Answer from the drawing. Dimensions are ordinates in mm from the lowest x, y and z of the part. A direction names the side the tool comes from. Coordinates: 2 decimals unless noted, no trailing zeros. Write each loop counter-clockwise with the first axis right and the second up, starting at its lowest first coordinate (ties: lowest second). Pieces come first, ordered by that corner, then holes. Notation, with made-up numbers: (-39.75, -35) - (-34.75, -35) arc R15 cw to (-34.75, -24) - close; hole circle Ø10 at (78, 9.5). An arc over 180 degrees is marked (long way). Use a Markdown table: item, result.
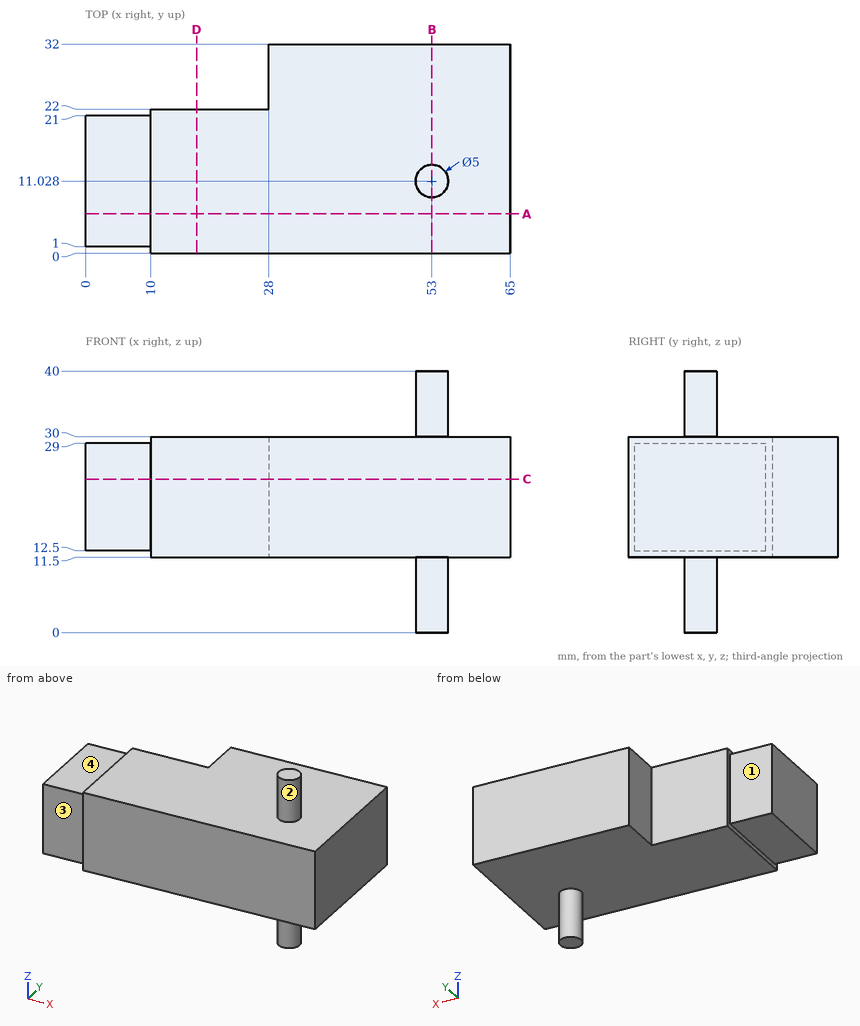
(1) A cutting plane is placed at C-C, the plane z = 23.5. Write down the section's boundary in (x, y), and give its area (3 significant figures).
Report:
| item | result |
|---|---|
| outline | (0, 1) - (10, 1) - (10, 0) - (65, 0) - (65, 32) - (28, 32) - (28, 22) - (10, 22) - (10, 21) - (0, 21) - close |
| area | 1,780 mm² |
(2) A cutting plane is placed at B-B, the plane x = 53. Write down the section's boundary in (y, z).
Report:
| item | result |
|---|---|
| outline | (0, 11.5) - (8.53, 11.5) - (8.53, 0) - (13.53, 0) - (13.53, 11.5) - (32, 11.5) - (32, 30) - (13.53, 30) - (13.53, 40) - (8.53, 40) - (8.53, 30) - (0, 30) - close |
(3) For the marked faces 1, 2, 3 and 4, determine the directions among +Z, -Z, +X, -X, +Y, -Y from which every point of the face is accessible in a straight line to the end or side of a thin tool.
Report:
| item | result |
|---|---|
| face 1 | +Z, -Z, -X, +Y |
| face 2 | +Z |
| face 3 | +Z, -Z, -X, -Y |
| face 4 | +Z, -X, +Y, -Y |
(4) A cutting plane is placed at D-D, the plane x = 17. Write down the section's boundary in (y, z).
Report:
| item | result |
|---|---|
| outline | (0, 11.5) - (22, 11.5) - (22, 30) - (0, 30) - close |
(5) Straight lines are drawn through the part: L1, parallel to Y at x = 17, z = 19; L2, parallel to Z at x = 32, y = 17.5; L3, parallel to X at y = 12.5, z = 12. For each, find the intervals that lie inside material, in ascending order.
Report:
| item | result |
|---|---|
| L1 | y = 0 to 22 |
| L2 | z = 11.5 to 30 |
| L3 | x = 10 to 65 |
(6) A cutting plane is placed at A-A, the plane y = 6. Write down the section's boundary in (x, z), and give its area (3 significant figures).
Report:
| item | result |
|---|---|
| outline | (0, 12.5) - (10, 12.5) - (10, 11.5) - (65, 11.5) - (65, 30) - (10, 30) - (10, 29) - (0, 29) - close |
| area | 1,180 mm² |
(7) Each of these flat-tipped pins is pushed along its axis until it touches: P1, Ø14.5, axis at x = 16, z = 25.5, coming from the +Y side; P2, Ø3, axis at x = 7, z = 18.5, coming from the +Y side; P3, Ø5, axis at x = 5.5, y = 11.5, coming from the +Z side. Where does it stop, or does it pass through?
Report:
| item | result |
|---|---|
| P1 | stops at y = 22 |
| P2 | stops at y = 21 |
| P3 | stops at z = 29 |
